For this review, take the finished solid that the model builds, in its own axes (mm). A direction names the side the tool comes from. Give positions to 0.01 mm unless a question says otherwise; leave off trailing zeros. Order: outer loops, then holes, each group sorted by start corner. A loop starts at its lowest first (then second) coordinate and runs counter-clockwise, first axis right, second up. Notation, with made-up numbers: (74, -14.5) -> (81, -14.5) arc R21 ccw to (81, 8.5) -> close; hole circle Ø7 at (-2, 63.5). An arc over 180 degrees is marked (long way). Return JSON: item names as keys, results as strings. Group by question number.
1) To check wall thickness, follow line 1 along X through (y, z) = (0.6, 0); line 2 along X through (y, z) = (0.35, 0); line 3 along Y through (x, z) = (-8.5, 6.6). State the ranges of each line that lie inside material, in increasing order.
2) For faces 1 (the face through (-7, 0.5, 1)), 2 (the face through (-31.5, 1, 2)), list the 3-axis set-ups (+Z, -Z, +X, -X, +Y, -Y) from which the entire face can be reached by the end or side of a thin tool; tool diameter is ignored.
3) Add section A-A (x = 27.5). Give the boundary of the cut face in (y, z).
4) Insertion check: P1, Ø3, axis at x = 6.5, y = 5.4, coming from the -Z side; P2, Ø4, axis at x = 6, y = 4.5, coming from the -Z side; P3, Ø1, axis at x = -25, z = -4, coming from the -Y side. Each pin has a flat end and moves straight along its axis. Give the tip position at first contact, or say it passes through.
5) The part is to be moulded in two halves that separate along Y. For faces 3 (the face through (18.677, 0.732, 2.769)), 4 (the face through (26, -2, 0)), 5 (the face through (-9, 4, 6.25)), 6 (the face through (-9.25, 4.82, 6.88)), say which applies: released by +Y, released by -Y, zero draft, split by the parting line, or undercut.
6) Add section B-B (z = 0). State how many separate pieces and enclosed holes the cut face has, then the cut area to 3 significant figures.
7) Add section C-C (x = -19.5). Give the boundary of the cut face in (y, z).
from build123d import *

# Parameters (mm, degrees)
SKETCH_1_W               = 48
SKETCH_1_H               = 15
SKETCH_1_R               = 1.1
SKETCH_1_R_2             = 1
SKETCH_1_R_3             = 1.5
SKETCH_1_R_4             = 2.5
EXTRUDE_1_DEPTH          = 2
EXTRUDE_2_DEPTH          = 2
SKETCH_4_R               = 3
CUT_EXTRUDE_1_DEPTH      = 1.5
SKETCH_5_W               = 46
SKETCH_5_H               = 1.5
EXTRUDE_3_DEPTH          = 5
SKETCH_2_3_R             = 0.95
CUT_EXTRUDE_2_DEPTH      = 6
CUT_EXTRUDE_START        = -0.25
SKETCH_7_R               = 0.95
CUT_EXTRUDE_3_DEPTH      = 0.25
SKETCH_1_3_W             = 15
SKETCH_1_3_H             = 15
SKETCH_1_3_R             = 6
SKETCH_1_3_R_2           = 1.5
SKETCH_1_3_R_3           = 1.1
EXTRUDE_4_DEPTH          = 2
EXTRUDE_START            = -2
SKETCH_1_4_W             = 15
SKETCH_1_4_H             = 15
SKETCH_1_4_R             = 6
SKETCH_1_4_R_2           = 1.5
SKETCH_1_4_R_3           = 1.1
EXTRUDE_5_DEPTH          = 2
CUT_EXTRUDE_4_DEPTH      = 2
CUT_EXTRUDE_4_DEPTH_BACK = 0.5
SKETCH_1_5_R             = 6
CUT_EXTRUDE_5_DEPTH      = 15
SKETCH_9_R               = 3.6
SKETCH_9_R_2             = 2.5
EXTRUDE_6_DEPTH          = 2


with BuildPart() as part:
    # 草图1 → 凸台-拉伸1 (new body)
    with BuildSketch(Plane(origin=(0, 0, 0), x_dir=(1, 0, 0), z_dir=(0, 1, 0))):
        with Locations((-7.5, 0)):
            Rectangle(SKETCH_1_W, SKETCH_1_H)
        with Locations(Location((-4.169872981, -2.5, 0), (0, 0, 270))):
            Circle(SKETCH_1_R, mode=Mode.SUBTRACT)
        with Locations(Location((3, 0, 0), (0, 0, 270))):
            Circle(SKETCH_1_R_2, mode=Mode.SUBTRACT)
        with Locations(Location((-8.5, 0, 0), (0, 0, 270))):
            Circle(SKETCH_1_R_3, mode=Mode.SUBTRACT)
        with Locations(Location((-12.830127019, 2.5, 0), (0, 0, 270))):
            Circle(SKETCH_1_R, mode=Mode.SUBTRACT)
        with Locations(Location((8, 0, 0), (0, 0, 270))):
            Circle(SKETCH_1_R_4, mode=Mode.SUBTRACT)
        with Locations(Location((13, 0, 0), (0, 0, 270))):
            Circle(SKETCH_1_R_2, mode=Mode.SUBTRACT)
        with Locations(Location((8, 5, 0), (0, 0, 270))):
            Circle(SKETCH_1_R_2, mode=Mode.SUBTRACT)
    extrude(amount=EXTRUDE_1_DEPTH)

    # 草图2 → 凸台-拉伸2 (add)
    with BuildSketch(Plane.XY.offset(7.5)):
        with BuildLine():
            Line((-22.1, 1.4), (-24.9, 1.4))
            ThreePointArc((-24.9, 1.4), (-23.5, 0), (-22.1, 1.4))
        make_face()
        with BuildLine():
            ThreePointArc((-24.764911064, 2), (-24.865810289, 1.707509764), (-24.9, 1.4))
            Line((-24.9, 1.4), (-22.1, 1.4))
            ThreePointArc((-22.1, 1.4), (-22.134189711, 1.707509764), (-22.235088936, 2))
            Line((-22.235088936, 2), (-24.764911064, 2))
        make_face()
        with BuildLine():
            ThreePointArc((-22.235088936, 2), (-23.5, 2.8), (-24.764911064, 2))
            Line((-24.764911064, 2), (-22.235088936, 2))
        make_face()
        with BuildLine():
            Line((-7.1, 1.4), (-9.9, 1.4))
            ThreePointArc((-9.9, 1.4), (-8.5, 0), (-7.1, 1.4))
        make_face()
        with BuildLine():
            ThreePointArc((-9.764911064, 2), (-9.865810289, 1.707509764), (-9.9, 1.4))
            Line((-9.9, 1.4), (-7.1, 1.4))
            ThreePointArc((-7.1, 1.4), (-7.134189711, 1.707509764), (-7.235088936, 2))
            Line((-7.235088936, 2), (-9.764911064, 2))
        make_face()
        with BuildLine():
            ThreePointArc((-7.235088936, 2), (-8.5, 2.8), (-9.764911064, 2))
            Line((-9.764911064, 2), (-7.235088936, 2))
        make_face()
        with BuildLine():
            Line((7.9, 1.4), (5.1, 1.4))
            ThreePointArc((5.1, 1.4), (6.5, 0), (7.9, 1.4))
        make_face()
        with BuildLine():
            ThreePointArc((5.235088936, 2), (5.134189711, 1.707509764), (5.1, 1.4))
            Line((5.1, 1.4), (7.9, 1.4))
            ThreePointArc((7.9, 1.4), (7.865810289, 1.707509764), (7.764911064, 2))
            Line((7.764911064, 2), (5.235088936, 2))
        make_face()
        with BuildLine():
            ThreePointArc((7.764911064, 2), (6.5, 2.8), (5.235088936, 2))
            Line((5.235088936, 2), (7.764911064, 2))
        make_face()
    extrude(amount=EXTRUDE_2_DEPTH)

    # 草图4 → 切除-拉伸1 (cut)
    with BuildSketch(Plane(origin=(0, 2, 0), x_dir=(1, 0, 0), z_dir=(0, 1, 0))):
        with Locations(Location((-8.5, 0, 0), (0, 0, 270))):
            Circle(SKETCH_4_R)
    extrude(amount=-CUT_EXTRUDE_1_DEPTH, mode=Mode.SUBTRACT)

    # 草图5 → 凸台-拉伸3 (add)
    with BuildSketch(Plane(origin=(0, 2, 0), x_dir=(1, 0, 0), z_dir=(0, 1, 0))):
        with Locations((-8.5, -6.75)):
            Rectangle(SKETCH_5_W, SKETCH_5_H)
    extrude(amount=EXTRUDE_3_DEPTH)

    # 草图2<3> → 切除-拉伸2 (cut)
    with BuildSketch(Plane.XY.offset(7.5)):
        with Locations((-23.5, 5.4)):
            Circle(SKETCH_2_3_R)
        with Locations((-8.5, 5.4)):
            Circle(SKETCH_2_3_R)
        with Locations((6.5, 5.4)):
            Circle(SKETCH_2_3_R)
    extrude(amount=-CUT_EXTRUDE_2_DEPTH, mode=Mode.SUBTRACT)

    # 草图7 → 切除-拉伸3 (cut)
    # profile 1 of 3: a face of its own
    with BuildSketch(Plane(origin=(0, 0, 6), x_dir=(-1, 0, 0), z_dir=(0, 0, -1)).offset(CUT_EXTRUDE_START)):
        Polygon((-7.596965511, 3.5), (-5.403034489, 3.5), (-4.306068977, 5.4), (-5.403034489, 7.3), (-7.596965511, 7.3), (-8.693931023, 5.4), align=None)
        with Locations(Location((-6.5, 5.4, 0), (0, 0, 180))):
            Circle(SKETCH_7_R, mode=Mode.SUBTRACT)
    # profile 2 of 3: a face of its own
    with BuildSketch(Plane(origin=(0, 0, 6), x_dir=(-1, 0, 0), z_dir=(0, 0, -1)).offset(CUT_EXTRUDE_START)):
        Polygon((6.306068977, 5.4), (7.403034489, 3.5), (9.596965511, 3.5), (10.693931023, 5.4), (9.596965511, 7.3), (7.403034489, 7.3), align=None)
        with Locations(Location((8.5, 5.4, 0), (0, 0, 180))):
            Circle(SKETCH_7_R, mode=Mode.SUBTRACT)
    # profile 3 of 3: a face of its own
    with BuildSketch(Plane(origin=(0, 0, 6), x_dir=(-1, 0, 0), z_dir=(0, 0, -1)).offset(CUT_EXTRUDE_START)):
        Polygon((21.306068977, 5.4), (22.403034489, 3.5), (24.596965511, 3.5), (25.693931023, 5.4), (24.596965511, 7.3), (22.403034489, 7.3), align=None)
    extrude(amount=CUT_EXTRUDE_3_DEPTH, mode=Mode.SUBTRACT)

    # 草图1<3> → 凸台-拉伸4 (add)
    # profile 1 of 2: a face of its own
    with BuildSketch(Plane(origin=(0, 0, 0), x_dir=(1, 0, 0), z_dir=(0, 1, 0))):
        with Locations((24, 0)):
            Rectangle(SKETCH_1_3_W, SKETCH_1_3_H)
        with Locations((24, 0)):
            Circle(SKETCH_1_3_R, mode=Mode.SUBTRACT)
    # profile 2 of 2: a face of its own
    with BuildSketch(Plane(origin=(0, 0, 0), x_dir=(1, 0, 0), z_dir=(0, 1, 0))):
        with Locations((24, 0)):
            Circle(SKETCH_1_3_R)
        with Locations(Location((24, 0, 0), (0, 0, 270))):
            Circle(SKETCH_1_3_R_2, mode=Mode.SUBTRACT)
        with Locations(Location((27.5, 0, 0), (0, 0, 270))):
            Circle(SKETCH_1_3_R_3, mode=Mode.SUBTRACT)
        with Locations(Location((24, -3.5, 0), (0, 0, 270))):
            Circle(SKETCH_1_3_R_3, mode=Mode.SUBTRACT)
        with Locations(Location((20.5, 0, 0), (0, 0, 270))):
            Circle(SKETCH_1_3_R_3, mode=Mode.SUBTRACT)
        with Locations(Location((24, 3.5, 0), (0, 0, 270))):
            Circle(SKETCH_1_3_R_3, mode=Mode.SUBTRACT)
    extrude(amount=EXTRUDE_4_DEPTH)

    # 草图1<4> → 凸台-拉伸5 (add)
    # profile 1 of 2: a face of its own
    with BuildSketch(Plane(origin=(0, 0, 0), x_dir=(1, 0, 0), z_dir=(0, 1, 0)).offset(EXTRUDE_START)):
        with Locations((24, 0)):
            Rectangle(SKETCH_1_4_W, SKETCH_1_4_H)
        with Locations((24, 0)):
            Circle(SKETCH_1_4_R, mode=Mode.SUBTRACT)
    # profile 2 of 2: a face of its own
    with BuildSketch(Plane(origin=(0, 0, 0), x_dir=(1, 0, 0), z_dir=(0, 1, 0)).offset(EXTRUDE_START)):
        with Locations((24, 0)):
            Circle(SKETCH_1_4_R)
        with Locations(Location((24, 0, 0), (0, 0, 270))):
            Circle(SKETCH_1_4_R_2, mode=Mode.SUBTRACT)
        with Locations(Location((27.5, 0, 0), (0, 0, 270))):
            Circle(SKETCH_1_4_R_3, mode=Mode.SUBTRACT)
        with Locations(Location((24, -3.5, 0), (0, 0, 270))):
            Circle(SKETCH_1_4_R_3, mode=Mode.SUBTRACT)
        with Locations(Location((20.5, 0, 0), (0, 0, 270))):
            Circle(SKETCH_1_4_R_3, mode=Mode.SUBTRACT)
        with Locations(Location((24, 3.5, 0), (0, 0, 270))):
            Circle(SKETCH_1_4_R_3, mode=Mode.SUBTRACT)
    extrude(amount=EXTRUDE_5_DEPTH)

    # 草图1<5> → 切除-拉伸4 (cut, two sides: drawn at the far end of the back side and taken through both)
    with BuildSketch(Plane(origin=(0, 0, 0), x_dir=(1, 0, 0), z_dir=(0, 1, 0)).offset(-CUT_EXTRUDE_4_DEPTH_BACK)):
        with Locations(Location((24, 0, 0), (0, 0, 270))):
            Circle(SKETCH_1_5_R)
    extrude(amount=CUT_EXTRUDE_4_DEPTH + CUT_EXTRUDE_4_DEPTH_BACK, mode=Mode.SUBTRACT)

    # 草图8 → 切除-拉伸5 (cut)
    with BuildSketch(Plane(origin=(0, 0, -7.5), x_dir=(-1, 0, 0), z_dir=(0, 0, -1))):
        Polygon((-16.5, 0), (-18.5, -2), (-16.5, -2), align=None)
    extrude(amount=-CUT_EXTRUDE_5_DEPTH, mode=Mode.SUBTRACT)

    # 草图9 → 凸台-拉伸6 (add)
    with BuildSketch(Plane(origin=(0, 2, 0), x_dir=(1, 0, 0), z_dir=(0, 1, 0))):
        with Locations(Location((8, 0, 0), (0, 0, 270))):
            Circle(SKETCH_9_R)
        with Locations(Location((8, 0, 0), (0, 0, 270))):
            Circle(SKETCH_9_R_2, mode=Mode.SUBTRACT)
    extrude(amount=EXTRUDE_6_DEPTH)


solid = part.part
Evaluation:
{
 "1": {"line 1": "-31.5 to -11.5, -5.5 to 2, 4 to 5.5, 10.5 to 12, 14 to 18, 30 to 31.5", "line 2": "-31.5 to -10, -7 to 2, 4 to 5.5, 10.5 to 12, 14 to 18, 30 to 31.5", "line 3": "0 to 4.45, 6.35 to 7"},
 "2": {"face 1": "+Y", "face 2": "+Z, -Z, -X, +Y, -Y"},
 "3": {"outline": "(-2, -7.5) -> (2, -7.5) -> (2, -4.87) -> (-0.5, -4.87) -> (-0.5, -1.1) -> (-2, -1.1) -> close; (-2, 1.1) -> (-0.5, 1.1) -> (-0.5, 4.87) -> (2, 4.87) -> (2, 7.5) -> (-2, 7.5) -> close"},
 "4": {"P1": "z = -3.47", "P2": "z = -3.6", "P3": "y = 0"},
 "5": {"face 3": "zero draft", "face 4": "released by -Y", "face 5": "undercut", "face 6": "undercut"},
 "6": {"separate pieces": "8", "enclosed holes": "0", "area": "88.8 mm^2"},
 "7": {"outline": "(0, -7.5) -> (2, -7.5) -> (2, 6) -> (7, 6) -> (7, 7.5) -> (0, 7.5) -> close"}
}
